Study the drawing (mm; zero at the part's minimum x, y, z) and answer. A direction names the side the tool comes from. Round coordinates to 2 decimals unless told otherwise and drop trailing zeros. Loops run counter-clockwise (first coordinate to the right, second up) from the corner with the lowest first, then second, coordinate; pieces in that order, holes last. Notation, with made-up numbers: (69.25, 76) - (85.25, 76) arc R18 cw to (85.25, 101) - close; hole circle Ø8 at (-1.5, 44.25). An arc over 180 degrees is marked (long way). Use CSV: the item, a comma, the result in double quotes. Start each with the question number.
1. Given pin 1 Ø9.5 at (x, y) = (137.75, 26.25) entering from +Z; pin 2 Ø5 at (x, z) = (138, 19) entering from +Y; pin 3 Ø3 at (x, z) = (4.5, 20.5) entering from +Y; pin 4 Ø15 at (x, z) = (43.5, 20.5) entering from +Y, each flat-ended and moving along its own axis, determine where each tip first touches the part or whether it passes through.
2. Find section D-D (x = 137). Give the vertices of the cut face in (y, z), and give its area (3 significant figures).
3. Find section A-A (z = 15). Give the vertices of the cut face in (x, y), and give its area (3 significant figures).
4. Determine the mould class of the marked faces 4, 5 and 6 for opening direction X: +X half, -X half, draft (parallel to the pull), parting line (faces both ways), or undercut.
5. Find section C-C (y = 13.5). Give the vertices of the cut face in (x, z), and give its area (3 significant figures).
6. A tool of negligible diameter and unlimited length cuts with its end or side. For the marked faces 1, 2 and 3, from which of +Z, -Z, +X, -X, +Y, -Y can it reach the whole face along a straight path? Write none if from no direction.
7. Consider line 1 along X through (y, z) = (3.65, 15); line 2 along X through (y, z) = (26.25, 26.4); line 3 along X through (y, z) = (31, 3.75). Determine where each line is inside the solid, lowest interval first.
8. Find section B-B (z = 4.75). Give the vertices of the cut face in (x, y), and give its area (3 significant figures).
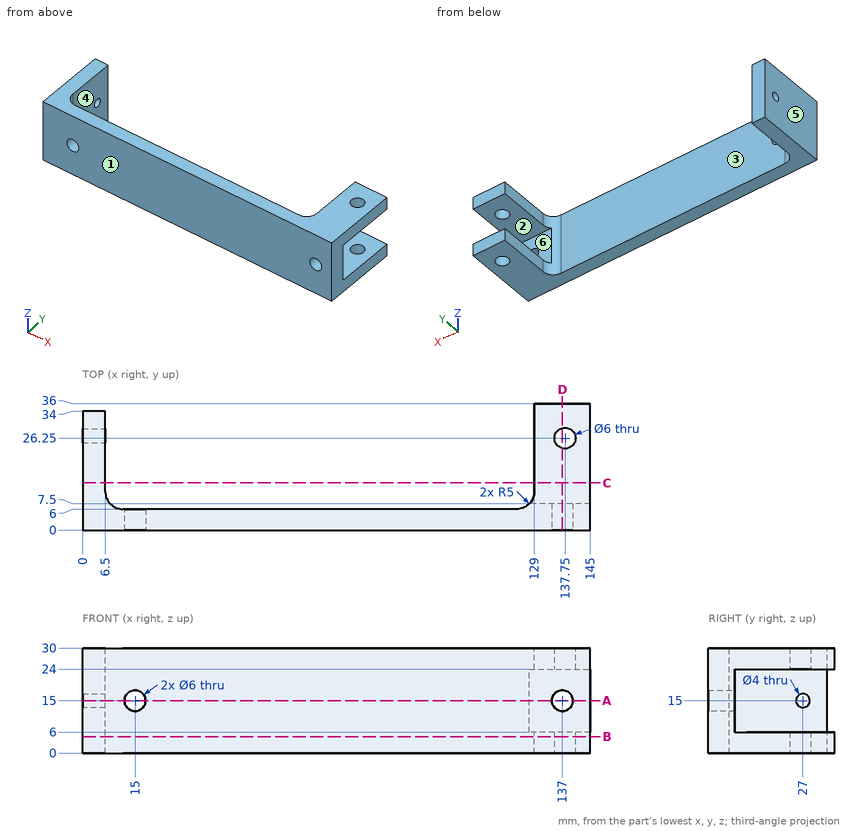
Filled sheet:
1,pin 1,"stops at z = 30"
1,pin 2,"stops at y = 7.5"
1,pin 3,"stops at y = 34"
1,pin 4,"stops at y = 6"
2,outline,"(0, 0) - (23.35, 0) - (23.35, 6) - (7.5, 6) - (7.5, 12) - (0, 12) - close; (0, 18) - (7.5, 18) - (7.5, 24) - (23.35, 24) - (23.35, 30) - (0, 30) - close; (29.15, 0) - (36, 0) - (36, 6) - (29.15, 6) - close; (29.15, 24) - (36, 24) - (36, 30) - (29.15, 30) - close"
2,area,"452 mm²"
3,outline,"(0, 0) - (12, 0) - (12, 6) - (11.5, 6) arc R5 cw to (6.5, 11) - (6.5, 25) - (0, 25) - close; (0, 29) - (6.5, 29) - (6.5, 34) - (0, 34) - close; (18, 0) - (134, 0) - (134, 7.5) - (127.57, 7.5) arc R5 cw to (124, 6) - (18, 6) - close; (140, 0) - (145, 0) - (145, 7.5) - (140, 7.5) - close"
3,area,"978 mm²"
4,face 4,"undercut"
4,face 5,"-X half"
4,face 6,"draft"
5,outline,"(0, 0) - (6.5, 0) - (6.5, 30) - (0, 30) - close; (129, 0) - (145, 0) - (145, 6) - (129, 6) - close; (129, 24) - (145, 24) - (145, 30) - (129, 30) - close"
5,area,"387 mm²"
6,face 1,"+Z, -Z, +X, -X, -Y"
6,face 2,"+X, +Y"
6,face 3,"+Z, -Z, +Y"
7,line 1,"x = 0 to 12, 18 to 134, 140 to 145"
7,line 2,"x = 0 to 6.5, 129 to 134.75, 140.75 to 145"
7,line 3,"x = 0 to 6.5, 129 to 145"
8,outline,"(0, 0) - (145, 0) - (145, 36) - (129, 36) - (129, 11) arc R5 cw to (124, 6) - (11.5, 6) arc R5 cw to (6.5, 11) - (6.5, 34) - (0, 34) - close; hole circle Ø6 at (137.75, 26.25)"
8,area,"1,510 mm²"
